Geometry check sheet. Reference: the model listing, model coordinates, mm. A direction names the side the tool comes from. Give positions to 0.01 mm unless a question says otherwise; leave off trailing zeros. Loops run counter-clockwise (first coordinate to the right, second up) from the corner with the lowest first, then second, coordinate; pieces in that order, holes last. Notation, with made-up numbers: (-31.5, 53) - (10.5, 53) arc R23 ccw to (10.5, 68) - close; hole circle Ø10 at (39.25, -2). An arc over 180 degrees is marked (long way). Use a Markdown table: item, result. Add a question column.
1. Material ranges on L1, parallel to X at y = 25, z = 0.5; L2, parallel to X at y = 20.5, z = 6.5; L3, parallel to Z at x = -18.5, y = 7, recorded low to high.
2. Cross-section at D-D on x = -10.5. Enter the section's corners in (y, z).
3. Draft check along Z on faces 1 (the flat face through (-12, 18, 3)), 2 (the flat face through (-20, 17.5, 2.8)), 3 (the flat face through (-11.6, 5.5, 4.25)), 4 (the flat face through (-10, 18, 10.2)). Enter one of: pulls with the +Z half, pulls with the -Z half, needs draft (parallel to the pull), parting line crosses it, or undercut.
4. Set-up check for faces 5 (the flat face through (-12, 30, 4.25)), 6 (the flat face through (-27.329, 17.452, -1.504)): record each of +Z, -Z, +X, -X, +Y, -Y from which the full face is reachable in a straight line by a thin tool's end or side.
5. Cross-section at A-A on z = 3.75. Enter the section's corners in (x, y), and give its area (3 significant figures).
6. Cross-section at B-B on y = 15.5. Enter the section's corners in (x, z).
7. Cross-section at C-C on x = -4.5. Enter the section's corners in (y, z).
8. Depth check by flat-ended pin: P1, Ø5, axis at x = -27.5, y = 19.5, coming from the -Z side; P2, Ø1.4, axis at x = -7.5, z = 3.5, coming from the -Y side; P3, Ø0.5, axis at x = -15.5, y = 29.5, coming from the -Z side; P4, Ø12, axis at x = -6.5, y = 5.5, coming from the -Z side. Enter the tip coordinate at first touch or a pass-through.
from build123d import *

# Parameters (mm, degrees)
F0_W     = 20
F0_H     = 35.4
F1_DEPTH = 10.2
F3_DEPTH = 17
F5_DEPTH = 35.4


with BuildPart() as f1:
    # F0 (on Top) → F1 (new body)
    with BuildSketch(Plane.XY):
        with Locations((-10, 17.7)):
            Rectangle(F0_W, F0_H)
    extrude(amount=F1_DEPTH)

    # F2 (on face) → F3 (cut)
    with BuildSketch(Plane(origin=(-20, 0, 0), x_dir=(0, -1, 0), z_dir=(-1, 0, 0))):
        Polygon((-5, 5.95), (-5, 7.2), (-30.4, 7.2), (-30.4, 5.95), (-29.4, 5.95), (-29.4, 4.25), (-30.4, 4.25), (-30.4, 3), (-5, 3), (-5, 4.25), (-6, 4.25), (-6, 5.95), align=None)
    extrude(amount=-F3_DEPTH, mode=Mode.SUBTRACT)

    # F4 (on face) → F5 (join)
    with BuildSketch(Plane.XZ):
        Polygon((-34.866854, -3.05), (0, 0), (-20, 0), align=None)
    extrude(amount=-F5_DEPTH)


solid = f1.part
Values found:
| question | item | result |
|---|---|---|
| 1 | L1 | x = -20 to 0 |
| 1 | L2 | x = -3 to 0 |
| 1 | L3 | z = -1.62 to 3, 7.2 to 10.2 |
| 2 | outline | (0, -0.92) - (35.4, -0.92) - (35.4, 10.2) - (0, 10.2) - close; hole (5, 3) - (30.4, 3) - (30.4, 4.25) - (29.4, 4.25) - (29.4, 5.95) - (30.4, 5.95) - (30.4, 7.2) - (5, 7.2) - (5, 5.95) - (6, 5.95) - (6, 4.25) - (5, 4.25) - close |
| 3 | face 1 | undercut |
| 3 | face 2 | needs draft |
| 3 | face 3 | undercut |
| 3 | face 4 | pulls with the +Z half |
| 4 | face 5 | -X |
| 4 | face 6 | +Z, -X, +Y, -Y |
| 5 | outline | (-20, 0) - (0, 0) - (0, 35.4) - (-20, 35.4) - (-20, 30.4) - (-3, 30.4) - (-3, 5) - (-20, 5) - close |
| 5 | area | 276 mm2 |
| 6 | outline | (-34.87, -3.05) - (0, 0) - (0, 10.2) - (-20, 10.2) - (-20, 7.2) - (-3, 7.2) - (-3, 3) - (-20, 3) - (-20, 0) - close |
| 7 | outline | (0, -0.39) - (35.4, -0.39) - (35.4, 10.2) - (0, 10.2) - close; hole (5, 3) - (30.4, 3) - (30.4, 4.25) - (29.4, 4.25) - (29.4, 5.95) - (30.4, 5.95) - (30.4, 7.2) - (5, 7.2) - (5, 5.95) - (6, 5.95) - (6, 4.25) - (5, 4.25) - close |
| 8 | P1 | stops at z = -2.62 |
| 8 | P2 | stops at y = 0 |
| 8 | P3 | stops at z = -1.38 |
| 8 | P4 | stops at z = -1.09 |
